Work out the finished part from the listing and answer in its coordinate system (mm). A direction names the side the tool comes from. Round coordinates to 2 decimals unless told otherwise and drop trailing zeros. Order: outer loops, then holes, each group sorted by start corner. A loop starts at its lowest first (then second) coordinate and runs counter-clockwise, first axis right, second up. Notation, with made-up numbers: M -18,55 L 32,55 A23 ccw 32,70 Z; hole C 55.5,37 d7. An arc over 180 degrees is marked long. Answer as a JSON object with one key per item and string values. Group by question number.
from build123d import *

# Parameters (mm, degrees)
F0_R     = 38.095
F0_R_2   = 17.08
F1_DEPTH = 28.6
F0_R_3   = 100
F2_DEPTH = 6.5
F0_R_4   = 114
F3_DEPTH = 20.5
F4_SIZE  = 13.99999
F0_R_5   = 124
F5_DEPTH = 20.5


# Not quite as in the source:
# - a fillet or chamfer is up to 0.001 mm smaller than in the source, because OpenCascade refuses the exact size


with BuildPart() as f1:
    # F0 (on Front) → F1 (new body, symmetric)
    with BuildSketch(Plane.XZ):
        Circle(F0_R)
        Circle(F0_R_2, mode=Mode.SUBTRACT)
    extrude(amount=F1_DEPTH, both=True)

    # F0 (on Front) → F2 (join, symmetric)
    with BuildSketch(Plane.XZ):
        Circle(F0_R_3)
        with BuildLine():
            Line((-57.3000000001, -75.7740720829), (-14.84, -37.9464020034))
            ThreePointArc((-14.84, -37.9464020034), (-0.0346057341, -40.7449853042), (14.775520982, -37.9715552053))
            Line((14.775520982, -37.9715552053), (14.7748944579, -37.9464020034))
            Line((14.7748944579, -37.9464020034), (14.7947522966, -37.9640662928))
            Line((14.7947522966, -37.9640662928), (57.2999999977, -75.7740720847))
            ThreePointArc((57.2999999977, -75.7740720847), (-1.5e-09, -95.0000000002), (-57.3000000001, -75.7740720829))
        make_face(mode=Mode.SUBTRACT)
        with BuildLine():
            Line((75.7740720829, -57.3), (37.9464020034, -14.84))
            ThreePointArc((37.9464020034, -14.84), (40.7449927617, -0.0242867339), (37.9640662928, 14.7947522966))
            Line((37.9640662928, 14.7947522966), (75.7740720847, 57.2999999977))
            ThreePointArc((75.7740720847, 57.2999999977), (95.0000000002, -1.5e-09), (75.7740720829, -57.3))
        make_face(mode=Mode.SUBTRACT)
        with BuildLine():
            ThreePointArc((-75.7740720847, -57.2999999977), (-95.0000000002, 1.5e-09), (-75.7740720829, 57.3000000001))
            Line((-75.7740720829, 57.3), (-37.9464020034, 14.84))
            ThreePointArc((-37.9464020034, 14.84), (-40.7449927617, 0.0242867339), (-37.9640662928, -14.7947522966))
            Line((-37.9640662928, -14.7947522966), (-75.7740720847, -57.2999999977))
        make_face(mode=Mode.SUBTRACT)
        Circle(F0_R, mode=Mode.SUBTRACT)
        with BuildLine():
            Line((57.3, 75.7740720829), (14.84, 37.9464020034))
            ThreePointArc((14.84, 37.9464020034), (0.0242867339, 40.7449927617), (-14.7947522966, 37.9640662928))
            Line((-14.7947522966, 37.9640662928), (-57.2999999977, 75.7740720847))
            ThreePointArc((-57.2999999977, 75.7740720847), (1.5e-09, 95.0000000002), (57.3, 75.7740720829))
        make_face(mode=Mode.SUBTRACT)
    extrude(amount=F2_DEPTH, both=True)

    # F0 (on Front) → F3 (join, symmetric)
    with BuildSketch(Plane.XZ):
        Circle(F0_R_4)
        Circle(F0_R_3, mode=Mode.SUBTRACT)
    extrude(amount=F3_DEPTH, both=True)

    # F4 (size 14 in the source; OpenCascade refuses exactly that, so slightly less here)
    f4_edges = [f1.edges().sort_by_distance(p)[0] for p in [
        (-100, -20.5, 0),
        (-100, 20.5, 0),
    ]]
    chamfer(f4_edges, length=F4_SIZE)

    # F0 (on Front) → F5 (join, symmetric)
    with BuildSketch(Plane.XZ):
        Circle(F0_R_5)
        Circle(F0_R_4, mode=Mode.SUBTRACT)
    extrude(amount=F5_DEPTH, both=True)


solid = f1.part
Item 1: Find section D-D (y = -13). Give the vertices of the cut face in (x, z) (3 decimals).
Item 2: Find section B-B (z = 0). Give the number of separate pieces and of enclosed holes in the cut face, and give its area (3 significant figures).
Item 3: A tool of negligible diameter and unlimited length cuts with its end or side. For faces 1 (the conical face through (-79.9, 7.18, -61.26)), 2 (the flat face through (14, -6.5, -37)), 3 (the cylindrical face through (40.744, 0.091, -0.237)), from which of +Z, -Z, +X, -X, +Y, -Y can it reach the whole face along a straight path? Write none if from no direction.
Item 4: Consider L1, parallel to Z at x = 34.5, y = 11.5; L2, parallel to Z at x = 0, y = -11 (3 decimals); L3, parallel to Z at x = 0, y = -7 (3 decimals). Determine where each line is inside the solid, lowest interval first.
Item 5: Find section A-A (y = 0). Give the vertices of the cut face in (x, z) (3 decimals), and give its area (3 significant figures).
Item 6: Each of these flat-tipped pins is pushed along its axis until it touches: pin 1 (4 mm diameter, centred on x = 63, z = -40.5, fed in from -Y); pin 2 (1.5 mm diameter, centred on x = 30.5, y = 15.5, fed in from +Z); pin 3 (2 mm diameter, centred on y = 15.5, z = -50.5, fed in from +X). Where does it stop, or does it pass through?
Item 7: The mould has two halves that part along Z. Classify faces 4 (the flat face through (100.5, -20.5, -54.5)), 5 (the flat face through (36.37, 0.09, 57.13)): +Z half, -Z half, draft (parallel to the pull), parting line (faces both ways), or undercut.
Responses:
{
 "1": {"outline": "C 0,0 d248; C 0,0 d76.19; hole C 0,0 d213; hole C 0,0 d34.16"},
 "2": {"separate pieces": "4", "enclosed holes": "0", "area": "4,180 mm^2"},
 "3": {"face 1": "+Y", "face 2": "-Y", "face 3": "+Y, -Y"},
 "4": {"L1": "z = -119.1 to -99.17, -16.15 to 16.15, 99.17 to 119.1", "L2": "z = -124 to -104.5, -38.095 to -17.08, 17.08 to 38.095, 104.5 to 124", "L3": "z = -124 to -100.5, -38.095 to -17.08, 17.08 to 38.095, 100.5 to 124"},
 "5": {"outline": "C 0,0 d248; hole M -75.774,-57.3 L -37.964,-14.795 A40.745 cw -37.946,14.84 L -75.774,57.3 A95 ccw Z; hole M -57.3,-75.774 A95 ccw 57.3,-75.774 L 14.775,-37.946 L 14.776,-37.972 A40.745 cw -14.84,-37.946 Z; hole M -57.3,75.774 L -14.795,37.964 A40.745 cw 14.84,37.946 L 57.3,75.774 A95 ccw Z; hole C 0,0 d34.16; hole M 37.946,-14.84 L 75.774,-57.3 A95 ccw 75.774,57.3 L 37.964,14.795 A40.745 cw Z", "area": "30,700 mm^2"},
 "6": {"pin 1": "stops at y = -6.5", "pin 2": "stops at z = 120.38", "pin 3": "stops at x = 113.69"},
 "7": {"face 4": "draft", "face 5": "undercut"}
}
